from build123d import *

# Parameters (mm, degrees)
F0_R     = 4.025
F1_DEPTH = 15
F2_W     = 4
F2_H     = 8.8454233903
F2_H_2   = 9.964544284
F3_DEPTH = 28.6711009125
F4_W     = 4
F4_H     = 9.9010998965
F5_DEPTH = 7
F7_DEPTH = 29.7172600886


# Not quite as in the source:
# - a feature names something its author has since deleted; it is built from what else it names


with BuildPart() as f1:
    # F0 (on Front) → F1 (new body)
    with BuildSketch(Plane.XZ):
        with BuildLine():
            Line((15, -11.0706584528), (15, 20))
            Line((15, 20), (0, 20))
            Line((0, 20), (0, 6.8212319165))
            Line((0, 6.8212319165), (-14.6675774532, -14.7143399477))
            ThreePointArc((-14.6675774532, -14.7143399477), (-14.7123164503, -14.8254204168), (-14.7066683885, -14.9450387593))
            Line((-14.7066683885, -14.9450387593), (-14.5789844453, -15.4207687435))
            ThreePointArc((-14.5789844453, -15.4207687435), (-13.0080916481, -16.8695228666), (-11.0253572607, -16.0724299998))
            Line((-11.0253572607, -16.0724299998), (-5.025187618, -10.5899751145))
            ThreePointArc((-5.025187618, -10.5899751145), (-1.6056896263, -10.7821354433), (-1.6008698149, -14.2070250586))
            Line((-1.6008698149, -14.2070250586), (-8.307190612, -21.5265534699))
            Line((-8.307190612, -21.5265534699), (-8.307190612, -22.085826844))
            Line((-8.307190612, -22.085826844), (7.8228749335, -22.085826844))
            ThreePointArc((7.8228749335, -22.085826844), (12.9859504737, -17.8510774103), (15, -11.4844412258))
            Line((15, -11.4844412258), (15, -11.0706584528))
        make_face()
        with Locations((4.5535718091, -7.0535713993)):
            Circle(F0_R, mode=Mode.SUBTRACT)
    extrude(amount=F1_DEPTH)

    # F2 (on face) → F3 (cut, through all)
    with BuildSketch(Plane(origin=(-3.1736560215, 0, 2.1615328257), x_dir=(0, -1, 0), z_dir=(-0.8265088883, 0, 0.5629236693))):
        with Locations((7.5, -24.8409709683)):
            Rectangle(F2_W, F2_H)
        with Locations((7.5, -15.4359871311)):
            Rectangle(F2_W, F2_H_2)
    extrude(amount=-F3_DEPTH, mode=Mode.SUBTRACT)

    # F4 (on face) → F5 (cut)
    with BuildSketch(Plane(origin=(-3.1736560215, 0, 2.1615328257), x_dir=(0, -1, 0), z_dir=(-0.8265088883, 0, 0.5629236693))):
        with Locations((7.5, -5.5031650409)):
            Rectangle(F4_W, F4_H)
    extrude(amount=-F5_DEPTH, mode=Mode.SUBTRACT)

    # F6 (on face) → F7 (cut, through all)
    with BuildSketch(Plane.YZ.offset(15)):
        Polygon((-9.4687892124, -16.3104510802), (-9.4687892124, -22.085826844), (-5.6066988036, -22.085826844), (-5.6066988036, -16.3104510802), (-5.6066988036, -12.8443576396), (-9.4687892124, -12.8443576396), align=None)
    extrude(amount=-F7_DEPTH, mode=Mode.SUBTRACT)


solid = f1.part
Read the model definition and answer for the solid it produces. Units are mm, in the model's axes. A direction names the side the tool comes from. Give positions to 0.01 mm unless a question says otherwise; leave off trailing zeros. Write each loop counter-clockwise with the first axis right and the second up, starting at its lowest first coordinate (ties: lowest second). Pieces come first, ordered by that corner, then holes. Notation, with made-up numbers: (56.25, 75.25) -> (104.25, 75.25) arc R28 ccw to (104.25, 108.25) -> close; hole circle Ø6 at (-17, 78). An arc over 180 degrees is marked (long way). Answer as a JSON object with one key per item and string values. Group by question number.
1) Consider L1, parallel to Y at x = -6.5, z = -3; L2, parallel to Y at x = 13, z = -14; L3, parallel to Z at x = 2.5, y = -13.5. Determine where each line is inside the solid, lowest interval first. Write a range as from..to.
2) Find section C-C (y = -6.5). Write down the section's boundary in (x, z) (3 decimals).
3) A tool of negligible diameter and unlimited length cuts with its end or side. For faces 4 (the flat face through (-8.1, -12.2, -13.4)), 5 (the flat face through (-6, -5.5, -6)), 6 (the flat face through (8, -8, -12.844)), from which of +Z, -Z, +X, -X, +Y, -Y can it reach the whole face along a straight path? Write none if from no direction.
4) Find section B-B (z = -5). Write down the section's boundary in (x, y).
5) The mould has two halves that part along Y. Classify faces 1 (the flat face through (9, -5.607, -16)), 2 (the flat face through (3, 0, -1)), 3 (the cylindrical face through (3.681, -7.395, -10.983)): +Y half, -Y half, draft (parallel to the pull), parting line (faces both ways), or undercut.
6) Find section D-D (x = 13.25). Write down the section's boundary in (y, z), and give its area (3 significant figures).
7) Each of these flat-tipped pins is pushed along its axis until it touches: P1, Ø1.2, axis at x = 4.5, y = -8, coming from the -Z side; P2, Ø0.6, axis at y = -2.5, z = -22, coming from the -X side. Where does it stop, or does it pass through?
Values follow:
{
 "1": {"L1": "y = -15..-9.5, -5.5..0", "L2": "y = -15..-9.47, -5.61..0", "L3": "z = -22.09..-10.52, -3.59..20"},
 "2": {"outline": "(-3.485, 1.705) -> (2.301, -2.236) -> (-3.012, -10.036) arc R2.495 cw to (-0.976, -11.983) -> (0.288, -12.844) -> (14.897, -12.844) arc R11.726 ccw to (15, -11.484) -> (15, 20) -> (0, 20) -> (0, 6.821) -> close; hole circle Ø8.05 at (4.554, -7.054)"},
 "3": {"face 4": "+Y, -Y", "face 5": "-X", "face 6": "-Z, +X, -X"},
 "4": {"outline": "(-8.05, -15) -> (1.09, -15) -> (1.09, 0) -> (-8.05, 0) -> (-8.05, -5.5) -> (0.42, -5.5) -> (0.42, -9.5) -> (-8.05, -9.5) -> close; (8.02, -15) -> (15, -15) -> (15, 0) -> (8.02, 0) -> close"},
 "5": {"face 1": "undercut", "face 2": "+Y half", "face 3": "draft"},
 "6": {"outline": "(-15, -17.44) -> (-9.47, -17.44) -> (-9.47, -12.84) -> (-5.61, -12.84) -> (-5.61, -17.44) -> (0, -17.44) -> (0, 20) -> (-15, 20) -> close", "area": "544 mm2"},
 "7": {"P1": "stops at z = -12.84", "P2": "stops at x = -8.31"}
}
